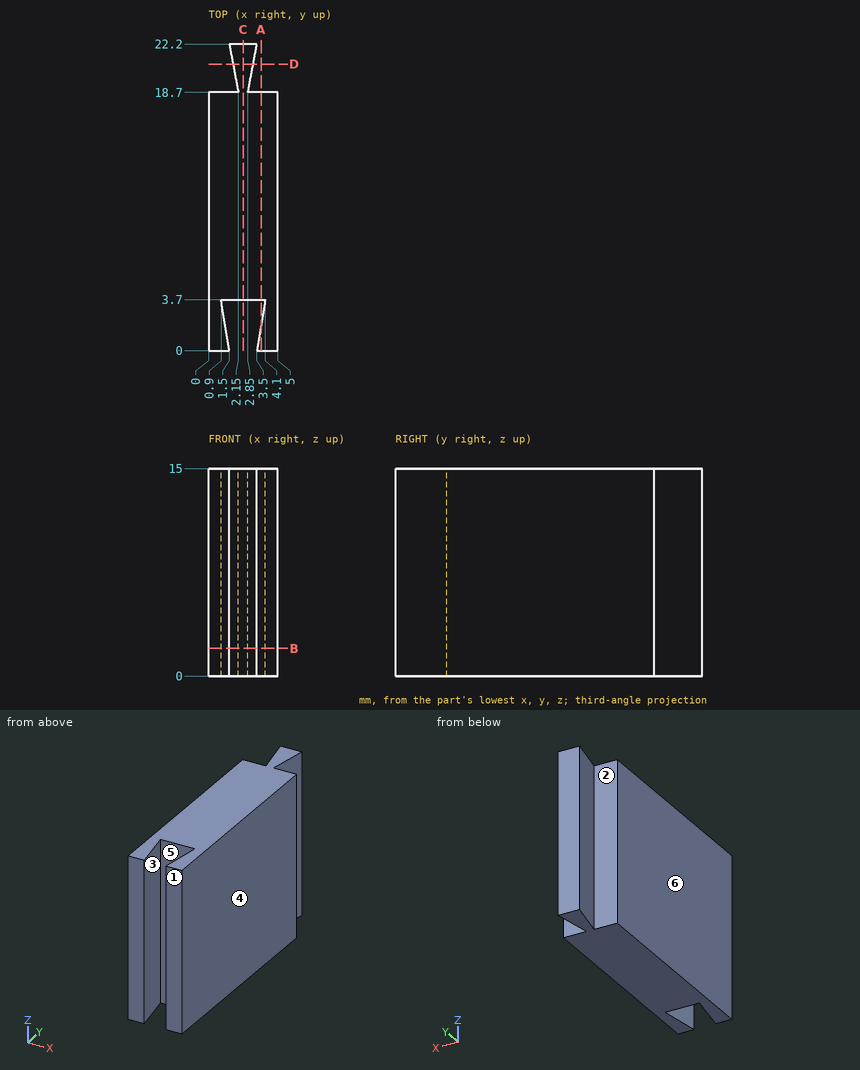
Geometry check sheet. Reference: drawing and pictorial views, mm from the part's lowest x, y, z. A direction names the side the tool comes from. Coordinates: 2 decimals unless noted, no trailing zeros. Order: outer loops, then holes, each group sorted by start corner. A loop starts at its lowest first (then second) coordinate and runs counter-clockwise, first axis right, second up.
Item 1: Section check C-C (x = 2.5). Enter the section's corners in (y, z).
Item 2: Section check B-B (z = 2). Enter the section's corners in (x, y), plus the area to 3 significant figures.
Item 3: Section check D-D (y = 20.75). Enter the section's corners in (x, z).
Item 4: Section check A-A (x = 3.8). Enter the section's corners in (y, z), plus the area to 3 significant figures.
Item 5: Mould release check, pull along X, two halves, no side actions. Record for the marked faces 4, 5 and 6: released by +X, released by -X, zero draft, split by the parting line, or undercut.
Item 6: Scan lines: line 1 along Y through (x, z) = (2.25, 1.25); line 2 along Y through (x, z) = (0.5, 8.25); line 3 along X through (y, z) = (1, 3.5). Record each from-to range of solid material in increasing order.
Item 7: Depth check by flat-ended pin: pin 1 (0.6 mm diameter, centred on x = 4.5, z = 10, fed in from +Y); pin 2 (3 mm diameter, centred on x = 1.5, y = 3, fed in from -Z); pin 3 (1.5 mm diameter, centred on x = 2.5, z = 10, fed in from -Y). Enter the tip coordinate at first touch or a pass-through.
Item 8: Tool access check on the marked faces 1, 2 and 3. Record the directions out of +Z, -Z, +X, -X, +Y, -Y that give a thin tool (end or side, any length) a straight path to the whole face; none if there is none.
Check sheet entries:
1. outline: (3.7, 0) - (22.2, 0) - (22.2, 15) - (3.7, 15) - close
2. outline: (0, 0) - (1.5, 0) - (0.9, 3.7) - (4.1, 3.7) - (3.5, 0) - (5, 0) - (5, 18.7) - (2.85, 18.7) - (3.5, 22.2) - (1.5, 22.2) - (2.15, 18.7) - (0, 18.7) - close
2. area: 88.6 mm2
3. outline: (1.77, 0) - (3.23, 0) - (3.23, 15) - (1.77, 15) - close
4. outline: (0, 0) - (1.85, 0) - (1.85, 15) - (0, 15) - close; (3.7, 0) - (18.7, 0) - (18.7, 15) - (3.7, 15) - close
4. area: 253 mm2
5. face 4: released by +X
5. face 5: undercut
5. face 6: released by -X
6. line 1: y = 3.7 to 22.2
6. line 2: y = 0 to 18.7
6. line 3: x = 0 to 1.34, 3.66 to 5
7. pin 1: stops at y = 18.7
7. pin 2: stops at z = 0
7. pin 3: stops at y = 3.7
8. face 1: +Z, -Z, +X, -X, -Y
8. face 2: +Z, -Z, -X
8. face 3: +Z, -Z
